from build123d import *

# Parameters (mm, degrees)
SKETCH_1_W          = 60
SKETCH_1_H          = 80
EXTRUDE_1_DEPTH     = 2
SKETCH_2_R          = 1.4
CUT_EXTRUDE_1_DEPTH = 50
SKETCH_3_R          = 2
CUT_EXTRUDE_2_DEPTH = 50
SKETCH_5_W          = 60
SKETCH_5_H          = 40
EXTRUDE_2_DEPTH     = 2
SKETCH_6_R          = 22
CUT_EXTRUDE_4_DEPTH = 50
SKETCH_4_R          = 1.65
CUT_EXTRUDE_3_DEPTH = 50
SKETCH_7_R          = 3
CUT_EXTRUDE_5_DEPTH = 14
SKETCH_8_R          = 1.6
CUT_EXTRUDE_6_DEPTH = 10
FILLET_1_R          = 10
CUT_EXTRUDE_7_DEPTH = 10
SKETCH_10_R         = 1.25
CUT_EXTRUDE_8_DEPTH = 10
SKETCH_11_W         = 43
SKETCH_11_H         = 7
CUT_EXTRUDE_9_DEPTH = 10
FILLET_2_R          = 2


with BuildPart() as part:
    # 草图1 → 凸台-拉伸1 (new body)
    with BuildSketch(Plane(origin=(0, 0, 0), x_dir=(1, 0, 0), z_dir=(0, 1, 0))):
        Rectangle(SKETCH_1_W, SKETCH_1_H)
    extrude(amount=EXTRUDE_1_DEPTH)

    # 草图2 → 切除-拉伸1 (cut)
    with BuildSketch(Plane(origin=(0, 2, 0), x_dir=(1, 0, 0), z_dir=(0, 1, 0))):
        with Locations(Location((0, -10.50070918, 0), (0, 0, 270))):
            Circle(SKETCH_2_R)
        with Locations(Location((9.49929082, -20, 0), (0, 0, 270))):
            Circle(SKETCH_2_R)
        with Locations(Location((0, -29.49929082, 0), (0, 0, 270))):
            Circle(SKETCH_2_R)
        with Locations(Location((-9.49929082, -20, 0), (0, 0, 270))):
            Circle(SKETCH_2_R)
    extrude(amount=-CUT_EXTRUDE_1_DEPTH, mode=Mode.SUBTRACT)

    # 草图3 → 切除-拉伸2 (cut)
    with BuildSketch(Plane(origin=(0, 2, 0), x_dir=(1, 0, 0), z_dir=(0, 1, 0))):
        with Locations(Location((0, -20, 0), (0, 0, 270))):
            Circle(SKETCH_3_R)
    extrude(amount=-CUT_EXTRUDE_2_DEPTH, mode=Mode.SUBTRACT)

    # 草图5 → 凸台-拉伸2 (add)
    with BuildSketch(Plane(origin=(0, 2, 0), x_dir=(1, 0, 0), z_dir=(0, 1, 0))):
        with Locations((0, 60)):
            Rectangle(SKETCH_5_W, SKETCH_5_H)
    extrude(amount=-EXTRUDE_2_DEPTH)

    # 草图6 → 切除-拉伸4 (cut)
    with BuildSketch(Plane(origin=(0, 2, 0), x_dir=(1, 0, 0), z_dir=(0, 1, 0))):
        with Locations(Location((0, 32, 0), (0, 0, 270))):
            Circle(SKETCH_6_R)
    extrude(amount=-CUT_EXTRUDE_4_DEPTH, mode=Mode.SUBTRACT)

    # 草图4 → 切除-拉伸3 (cut)
    with BuildSketch(Plane(origin=(0, 2, 0), x_dir=(1, 0, 0), z_dir=(0, 1, 0))):
        with Locations(Location((-7.5, 73.5, 0), (0, 0, 270))):
            Circle(SKETCH_4_R)
        with Locations(Location((7.5, 73.5, 0), (0, 0, 270))):
            Circle(SKETCH_4_R)
        with Locations(Location((7.5, 60.5, 0), (0, 0, 270))):
            Circle(SKETCH_4_R)
        with Locations(Location((-7.5, 60.5, 0), (0, 0, 270))):
            Circle(SKETCH_4_R)
    extrude(amount=-CUT_EXTRUDE_3_DEPTH, mode=Mode.SUBTRACT)

    # 草图7 → 切除-拉伸5 (cut)
    with BuildSketch(Plane(origin=(0, 2, 0), x_dir=(1, 0, 0), z_dir=(0, 1, 0))):
        with Locations(Location((0, -20, 0), (0, 0, 270))):
            Circle(SKETCH_7_R)
    extrude(amount=-CUT_EXTRUDE_5_DEPTH, mode=Mode.SUBTRACT)

    # 草图8 → 切除-拉伸6 (cut)
    with BuildSketch(Plane(origin=(0, 2, 0), x_dir=(1, 0, 0), z_dir=(0, 1, 0))):
        with Locations(Location((-25.5, 20, 0), (0, 0, 270))):
            Circle(SKETCH_8_R)
        with Locations(Location((-25.5, 5, 0), (0, 0, 270))):
            Circle(SKETCH_8_R)
        with Locations(Location((-25.5, -10, 0), (0, 0, 270))):
            Circle(SKETCH_8_R)
        with Locations(Location((-25.5, -25, 0), (0, 0, 270))):
            Circle(SKETCH_8_R)
        with Locations(Location((-25.5, 65, 0), (0, 0, 270))):
            Circle(SKETCH_8_R)
        with Locations(Location((-25.5, 50, 0), (0, 0, 270))):
            Circle(SKETCH_8_R)
        with Locations(Location((-25.5, 35, 0), (0, 0, 270))):
            Circle(SKETCH_8_R)
        with Locations(Location((25.5, 35, 0), (0, 0, 270))):
            Circle(SKETCH_8_R)
        with Locations(Location((25.5, 50, 0), (0, 0, 270))):
            Circle(SKETCH_8_R)
        with Locations(Location((25.5, 65, 0), (0, 0, 270))):
            Circle(SKETCH_8_R)
        with Locations(Location((25.5, -25, 0), (0, 0, 270))):
            Circle(SKETCH_8_R)
        with Locations(Location((25.5, -10, 0), (0, 0, 270))):
            Circle(SKETCH_8_R)
        with Locations(Location((25.5, 5, 0), (0, 0, 270))):
            Circle(SKETCH_8_R)
        with Locations(Location((25.5, 20, 0), (0, 0, 270))):
            Circle(SKETCH_8_R)
    extrude(amount=-CUT_EXTRUDE_6_DEPTH, mode=Mode.SUBTRACT)

    # 圆角1
    fillet_1_edges = [part.edges().sort_by_distance(p)[0] for p in [
        (-30, 1, -80),
        (30, 1, -80),
        (30, 1, 40),
        (-30, 1, 40),
    ]]
    fillet(fillet_1_edges, radius=FILLET_1_R)

    # 草图9 → 切除-拉伸7 (cut)
    with BuildSketch(Plane(origin=(0, 2, 0), x_dir=(1, 0, 0), z_dir=(0, 1, 0))):
        with BuildLine():
            ThreePointArc((-30, -30), (-27.963471357, -36.048398462), (-22.68337521, -39.633249581))
            ThreePointArc((-22.68337521, -39.633249581), (-28.111396766, -30.47613344), (-30, -20))
            Line((-30, -20), (-30, -30))
        make_face()
        with BuildLine():
            ThreePointArc((22.68337521, -39.633249581), (27.963471357, -36.048398462), (30, -30))
            Line((30, -30), (30, -20))
            ThreePointArc((30, -20), (28.111396766, -30.47613344), (22.68337521, -39.633249581))
        make_face()
    extrude(amount=-CUT_EXTRUDE_7_DEPTH, mode=Mode.SUBTRACT)

    # 草图10 → 切除-拉伸8 (cut)
    with BuildSketch(Plane(origin=(0, 2, 0), x_dir=(1, 0, 0), z_dir=(0, 1, 0))):
        with Locations(Location((-22.3, 75, 0), (0, 0, 270))):
            Circle(SKETCH_10_R)
        with Locations(Location((-25, 72.3, 0), (0, 0, 270))):
            Circle(SKETCH_10_R)
        with Locations(Location((25, 72.3, 0), (0, 0, 270))):
            Circle(SKETCH_10_R)
        with Locations(Location((22.3, 75, 0), (0, 0, 270))):
            Circle(SKETCH_10_R)
    extrude(amount=-CUT_EXTRUDE_8_DEPTH, mode=Mode.SUBTRACT)

    # 草图11 → 切除-拉伸9 (cut)
    with BuildSketch(Plane(origin=(0, 0, 0), x_dir=(-1, 0, 0), z_dir=(0, -1, 0))):
        with Locations((0, -2.5)):
            Rectangle(SKETCH_11_W, SKETCH_11_H)
    extrude(amount=-CUT_EXTRUDE_9_DEPTH, mode=Mode.SUBTRACT)

    # 圆角2
    fillet_2_edges = [part.edges().sort_by_distance(p)[0] for p in [
        (21.5, 1, 6),
        (21.5, 1, -1),
        (-21.5, 1, -1),
        (-21.5, 1, 6),
    ]]
    fillet(fillet_2_edges, radius=FILLET_2_R)


solid = part.part
Could you check a few things on this model? Use its own coordinates, in mm. Give positions to 0.01 mm unless a question says otherwise; leave off trailing zeros. Write each loop counter-clockwise with the first axis right and the second up, starting at its lowest first coordinate (ties: lowest second). Pieces come first, ordered by that corner, then holes. Notation, with made-up numbers: (28, 34) - (85, 34) arc R18 ccw to (85, 43) - close; hole circle Ø2 at (-4, -35). An arc over 180 degrees is marked (long way). Use CSV: the item, a comma, the result in double quotes. Start each with the question number.
Item 1: I want a section at A-A, the plane z = 2.5. Please give me the cut outline in (x, y), then the cut area to 3 significant figures.
Item 2: I want a section at C-C, the plane z = -20. Please give me the cut outline in (x, y).
Item 3: I want a section at B-B, the plane z = 25. Please give me the cut outline in (x, y), then the cut area to 3 significant figures.
Item 4: I want a section at D-D, the plane y = 1.45. Give the number of separate pieces and of enclosed holes in the cut face, then the cut area to 3 significant figures.
Item 5: If we mould it in two halves opening along X, with no side actions, what happens to faces 1 (the face through (25.05, 1.01, -73.55)), 2 (the face through (26.99, 0.99, -77.15))? For each: pulls with the +X half, pulls with the -X half, needs draft (parallel to the pull), parting line crosses it, or undercut.
Item 6: If I drill on line 1 along X through (y, z) = (1.25, 25); line 2 along Z through (x, y) = (2.5, 0.9); line 3 along Z through (x, y) = (-19.5, 1.55), over which ranges is the centre line in solid material (lowest first)?
Item 7: I'm going to push a flat-ended pin straight in: pin 1 (2 mm diameter, centred on x = -25, z = -72.3, fed in from +Y). Where does the tip first touch, or does it pass through?
Findings:
1,outline,"(-30, 0) - (-21.5, 0) - (-21.5, 2) - (-30, 2) - close; (21.5, 0) - (30, 0) - (30, 2) - (21.5, 2) - close"
1,area,"34.0 mm2"
2,outline,"(-30, 0) - (-27.1, 0) - (-27.1, 2) - (-30, 2) - close; (-23.9, 0) - (-18.44, 0) - (-18.44, 2) - (-23.9, 2) - close; (18.44, 0) - (23.9, 0) - (23.9, 2) - (18.44, 2) - close; (27.1, 0) - (30, 0) - (30, 2) - (27.1, 2) - close"
3,outline,"(-29.58, 0) - (-27.1, 0) - (-27.1, 2) - (-29.58, 2) - close; (-23.9, 0) - (23.9, 0) - (23.9, 2) - (-23.9, 2) - close; (27.1, 0) - (29.58, 0) - (29.58, 2) - (27.1, 2) - close"
3,area,"106 mm2"
4,separate pieces,"1"
4,enclosed holes,"29"
4,area,"5,020 mm2"
5,face 1,"undercut"
5,face 2,"pulls with the +X half"
6,line 1,"x = -29.58 to -27.1, -23.9 to 23.9, 27.1 to 29.58"
6,line 2,"z = -80 to -53.86, -10.14 to -1, 6 to 18.34, 21.66 to 40"
6,line 3,"z = -80 to -42.19, -21.81 to -1, 6 to 40"
7,pin 1,"passes through"
